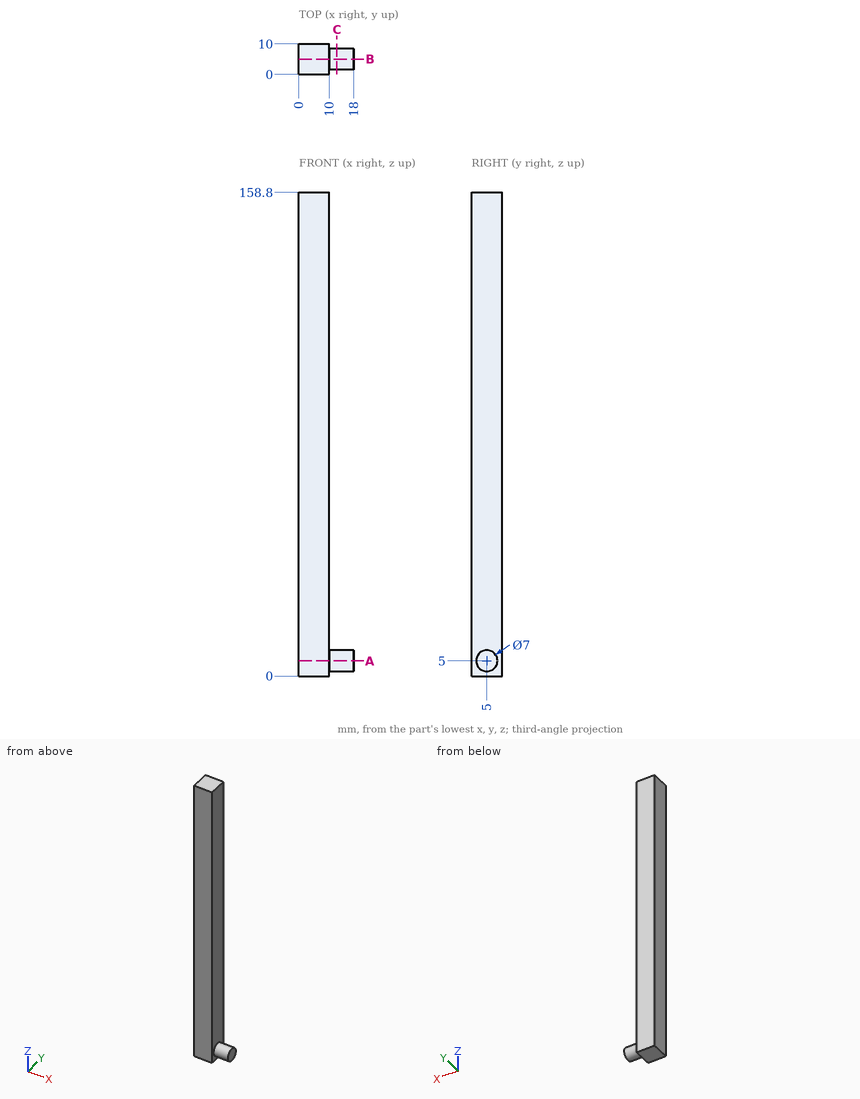
Design review of the part shown in the three views and the two pictorial views. Dimensions are in mm from the part's minimum x, y and z. Give positions to 0.01 mm unless a question says otherwise; leave off trailing zeros. Write each loop counter-clockwise with the first axis right and the second up, starting at its lowest first coordinate (ties: lowest second). Pieces come first, ordered by that corner, then holes.
(1) Add section B-B (y = 5). Give the boundary of the cut face in (x, z).
Checked values:
outline: (0, 0) - (10, 0) - (10, 1.5) - (18, 1.5) - (18, 8.5) - (10, 8.5) - (10, 158.8) - (0, 158.8) - close
(2) Add section A-A (z = 5). Give the boundary of the cut face in (x, y).
Checked values:
outline: (0, 0) - (10, 0) - (10, 1.5) - (18, 1.5) - (18, 8.5) - (10, 8.5) - (10, 10) - (0, 10) - close
(3) Add section C-C (x = 12.5). Give the boundary of the cut face in (y, z).
Checked values:
outline: circle Ø7 at (5, 5)
(4) Wall thickness on line 1 along X through (y, z) = (5, 89.5); line 2 along Z through (x, y) = (14, 5.25); line 3 along Z through (x, y) = (13.25, 2.25): over which ranges is each line inside the solid? List them lowest first.
Checked values:
line 1: x = 0 to 10
line 2: z = 1.51 to 8.49
line 3: z = 2.83 to 7.17
(5) Clearance check with flat-ended pins moving along their axes: pin 1 Ø10 at (x, z) = (14, 127) entering from -Y; pin 2 Ø5 at (y, z) = (5.5, 97) entering from +X; pin 3 Ø5 at (x, y) = (13.5, 2.5) entering from -Z. State where each tip first meets the part, or that it passes through.
Checked values:
pin 1: stops at y = 0
pin 2: stops at x = 10
pin 3: stops at z = 1.5
